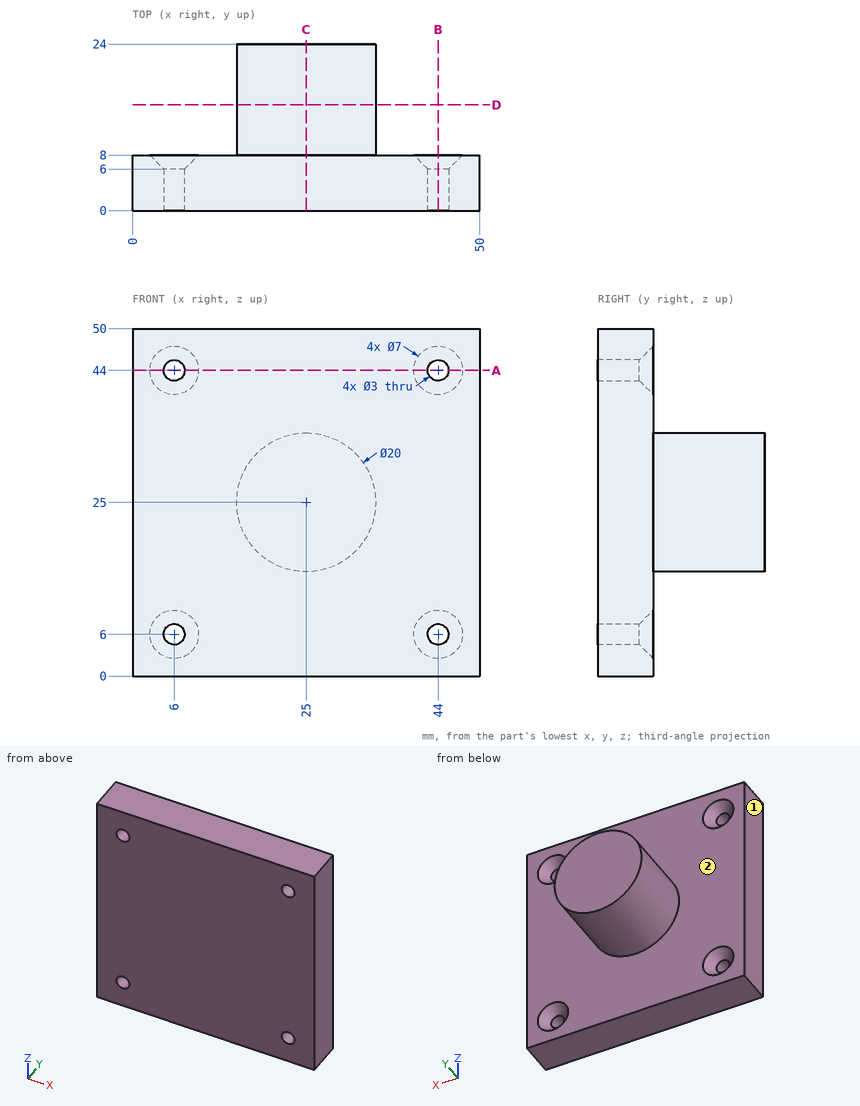
Could you check a few things on this drawing? It's one solid part, dimensions in mm from its lowest x, y, z. A direction names the side the tool comes from. Give positions to 0.01 mm unless a question says otherwise; leave off trailing zeros. Write each loop counter-clockwise with the first axis right and the second up, starting at its lowest first coordinate (ties: lowest second). Pieces come first, ordered by that corner, then holes.
(1) Imagine slicing it at B-B, the plane x = 44. Write out the boundary of the cut face in (y, z).
Output values:
outline: (0, 0) - (8, 0) - (8, 2.5) - (6, 4.5) - (0, 4.5) - close; (0, 7.5) - (6, 7.5) - (8, 9.5) - (8, 40.5) - (6, 42.5) - (0, 42.5) - close; (0, 45.5) - (6, 45.5) - (8, 47.5) - (8, 50) - (0, 50) - close
(2) Imagine slicing it at C-C, the plane x = 25. Write out the boundary of the cut face in (y, z).
Output values:
outline: (0, 0) - (8, 0) - (8, 15) - (24, 15) - (24, 35) - (8, 35) - (8, 50) - (0, 50) - close
(3) Imagine slicing it at A-A, the plane z = 44. Write out the boundary of the cut face in (x, y).
Output values:
outline: (0, 0) - (4.5, 0) - (4.5, 6) - (2.5, 8) - (0, 8) - close; (7.5, 0) - (42.5, 0) - (42.5, 6) - (40.5, 8) - (9.5, 8) - (7.5, 6) - close; (45.5, 0) - (50, 0) - (50, 8) - (47.5, 8) - (45.5, 6) - close
(4) On a 3-axis mill with a long thin cutter (end or side, diameter ignored), from which of +Z, -Z, +X, -X, +Y, -Y can I reach the whole of each face in a straight line? I mean the marked faces 1 and 2. Say none if no direction works.
Output values:
face 1: +Z, -Z, -X, +Y, -Y
face 2: +Y
(5) Imagine slicing it at D-D, the plane y = 15.25. Write out the boundary of the cut face in (x, z).
Output values:
outline: circle Ø20 at (25, 25)
(6) If I drill on L1, parallel to X at y = 3.9, z = 44; L2, parallel to Y at x = 10.5, z = 15.5, over which ranges is the centre line in solid material (lowest first)?
Output values:
L1: x = 0 to 4.5, 7.5 to 42.5, 45.5 to 50
L2: y = 0 to 8
(7) Will these pins go through, and if not, where does the flat tip stop? pin 1 (10 mm diameter, centred on y = 19, z = 42, fed in from -X); pin 2 (12 mm diameter, centred on y = 21, z = 10, fed in from +X); pin 3 (6 mm diameter, centred on x = 15.5, y = 13, fed in from -Z); pin 4 (3.5 mm diameter, centred on x = 6, z = 6, fed in from +Y).
Output values:
pin 1: passes through
pin 2: stops at x = 29.36
pin 3: stops at z = 17.4
pin 4: stops at y = 6.25
